from build123d import *

# Parameters (mm, degrees)
SKETCH1_R           = 19.05
SKETCH1_R_2         = 3.05
BOSS_EXTRUDE1_DEPTH = 1.27
BOSS_EXTRUDE2_DEPTH = 1.27
CIRPATTERN1_COUNT   = 4
BOSS_EXTRUDE3_DEPTH = 2.54


with BuildPart() as part:
    # Sketch1 → Boss-Extrude1 (new body)
    with BuildSketch(Plane.XY):
        Circle(SKETCH1_R)
        Circle(SKETCH1_R_2, mode=Mode.SUBTRACT)
    extrude(amount=BOSS_EXTRUDE1_DEPTH)

    # Sketch2 → Boss-Extrude2 (add)
    with BuildSketch(Plane(origin=(0, 0, 0), x_dir=(-1, 0, 0), z_dir=(0, 0, -1))):
        with BuildLine():
            Line((-1.524, 6.318815031), (-1.524, 7.588815031))
            Line((-1.524, 7.588815031), (1.524, 7.588815031))
            Line((1.524, 7.588815031), (1.524, 6.318815031))
            ThreePointArc((1.524, 6.318815031), (0, 6.499999954), (-1.524, 6.318815031))
        make_face()
    boss_extrude2 = extrude(amount=BOSS_EXTRUDE2_DEPTH)

    # CirPattern1: Boss-Extrude2 ×4 about axis
    cirpattern1_axis = Axis((0, 0, 0), (0, 0, 1))
    for i in range(1, CIRPATTERN1_COUNT):
        add(boss_extrude2.rotate(cirpattern1_axis, i * 360 / CIRPATTERN1_COUNT))

    # Sketch3 → Boss-Extrude3 (add, through all)
    with BuildSketch(Plane.XY.offset(1.27)):
        with BuildLine():
            Line((-1.673320053, 2.55), (1.673320053, 2.55))
            ThreePointArc((1.673320053, 2.55), (0, 3.05), (-1.673320053, 2.55))
        make_face()
    extrude(amount=-BOSS_EXTRUDE3_DEPTH)


solid = part.part
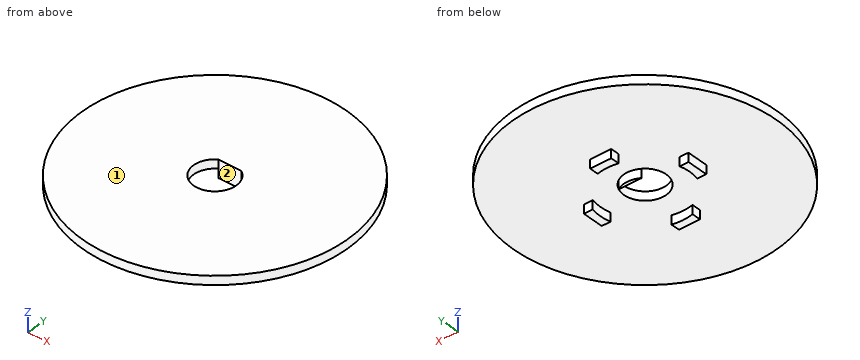
Build history of the part. All positions in model axes, mm. Face numbers are marked on the shaded views. Round coordinates to 2 decimals unless told otherwise and drop trailing zeros. Write each loop counter-clockwise with the first axis right and the second up, starting at its lowest first coordinate (ties: lowest second). Pieces come first, ordered by that corner, then holes. Notation, with made-up numbers: M 89,-33.5 L 107,-33.5 A23 ccw 107,-22.5 Z; hole C -32.75,-10.75 d9. An arc over 180 degrees is marked long. Answer as a JSON object with one key per item and string values. Group by question number.
(1) Cut at C-C (y = -10). Give the cut face in (x, z), and give its area (3 significant figures).
(2) Cut at D-D (x = 13). Give the cut face in (y, z).
(3) Cut at A-A (z = -0.65). Give the cut face in (x, y), and give its area (3 significant figures).
(4) Flat gauge pins, fed straight in: pin 1 (6 mm diameter, centred on x = -5, y = -15, fed in from -Z); pin 2 (0.6 mm diameter, centred on y = 7, z = -0.5, fed in from -X); pin 3 (1.4 mm diameter, centred on x = 0.5, z = -0.5, fed in from -Y). Where does each tip first touch, or does it go through?
(5) Cut at B-B (x = 0). Give the cut face in (y, z).
(6) Drill centre lines: L1, parallel to Y at x = 1, z = -1.05; L2, parallel to Y at x = 0, z = 0.55; L3, parallel to Z at x = -5, y = -11. Where is each one in solid material? Low to high.
(7) Mould opens along X. For the marked faces 1 and 2 say: pulls with the +X half, pulls with the -X half, needs draft (parallel to the pull), parting line crosses it, or undercut.
Responses:
{
 "1": {"outline": "M -16.21,0 L 16.21,0 L 16.21,1.27 L -16.21,1.27 Z", "area": "41.2 mm2"},
 "2": {"outline": "M -13.92,0 L 13.92,0 L 13.92,1.27 L -13.92,1.27 Z"},
 "3": {"outline": "M -7.59,-1.52 L -6.32,-1.52 A6.5 cw -6.32,1.52 L -7.59,1.52 Z; M -1.67,2.55 L 1.67,2.55 A3.05 ccw Z; M -1.52,-7.59 L 1.52,-7.59 L 1.52,-6.32 A6.5 cw -1.52,-6.32 Z; M -1.52,6.32 A6.5 cw 1.52,6.32 L 1.52,7.59 L -1.52,7.59 Z; M 6.32,-1.52 L 7.59,-1.52 L 7.59,1.52 L 6.32,1.52 A6.5 cw Z", "area": "15.1 mm2"},
 "4": {"pin 1": "stops at z = 0", "pin 2": "stops at x = -1.52", "pin 3": "stops at y = -19.05"},
 "5": {"outline": "M -19.05,0 L -7.59,0 L -7.59,-1.27 L -6.5,-1.27 L -6.5,0 L -3.05,0 L -3.05,1.27 L -19.05,1.27 Z; M 2.55,-1.27 L 3.05,-1.27 L 3.05,0 L 6.5,0 L 6.5,-1.27 L 7.59,-1.27 L 7.59,0 L 19.05,0 L 19.05,1.27 L 2.55,1.27 Z"},
 "6": {"L1": "y = -7.59 to -6.42, 2.55 to 2.88, 6.42 to 7.59", "L2": "y = -19.05 to -3.05, 2.55 to 19.05", "L3": "z = 0 to 1.27"},
 "7": {"face 1": "needs draft", "face 2": "undercut"}
}
